Verification items for this drawing (mm, ordinates from the low corner). Round coordinates to 2 decimals unless told otherwise and drop trailing zeros. Loops run counter-clockwise (first coordinate to the right, second up) from the corner with the lowest first, then second, coordinate; pieces in that order, holes last. Notation, with made-up numbers: (72, 8.5) - (122, 8.5) arc R30 cw to (122, 32.5) - close; hole circle Ø5 at (29, -11.75). An arc over 180 degrees is marked (long way). Answer in a Markdown table with one row per item. Add a question column.
(1) Cross-section at A-A on x = 1284.5. Enter the section's corners in (y, z), then the cut area to 3 significant figures.
(2) Cross-section at C-C on y = 37. Enter the section's corners in (x, z).
(3) Thickness scan on line 1 along Z through (x, y) = (1755, 32); line 2 along X through (y, z) = (31, 440). Record the ranges inside material, lowest first.
(4) Cross-section at B-B on z = 305.5. Enter the section's corners in (x, y).
(5) Cross-section at D-D on x = 310. Enter the section's corners in (y, z).
(6) Gauge pin test, flat ends, axial feed: pin 1 (12.5 mm diameter, centred on x = 299.5, y = 18.5, fed in from -Z); pin 2 (7.5 mm diameter, centred on y = 14, z = 964.5, fed in from +X); pin 3 (12.5 mm diameter, centred on y = 8, z = 961, fed in from -X). Record the tip position at first contact, or that the pin passes through.
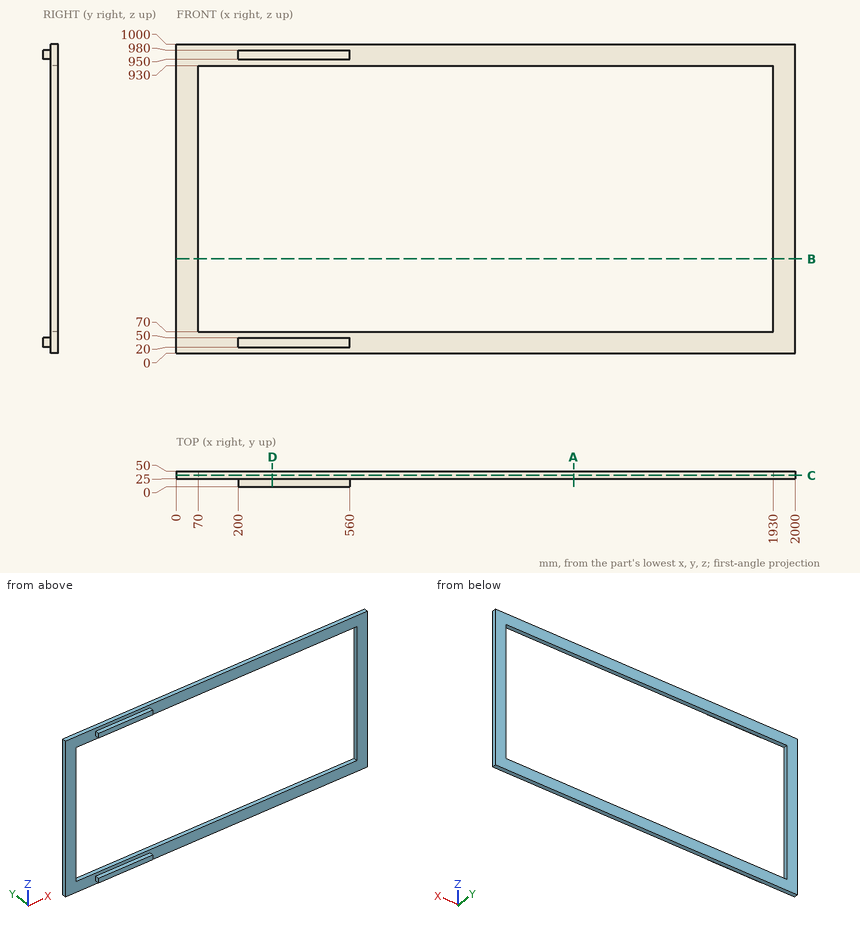
Answers:
| question | item | result |
|---|---|---|
| 1 | outline | (25, 0) - (50, 0) - (50, 70) - (25, 70) - close; (25, 930) - (50, 930) - (50, 1000) - (25, 1000) - close |
| 1 | area | 3,500 mm^2 |
| 2 | outline | (0, 0) - (2000, 0) - (2000, 1000) - (0, 1000) - close; hole (70, 70) - (1930, 70) - (1930, 930) - (70, 930) - close |
| 3 | line 1 | z = 0 to 70, 930 to 1000 |
| 3 | line 2 | x = 0 to 70, 1930 to 2000 |
| 4 | outline | (0, 25) - (70, 25) - (70, 50) - (0, 50) - close; (1930, 25) - (2000, 25) - (2000, 50) - (1930, 50) - close |
| 5 | outline | (0, 20) - (25, 20) - (25, 0) - (50, 0) - (50, 70) - (25, 70) - (25, 50) - (0, 50) - close; (0, 950) - (25, 950) - (25, 930) - (50, 930) - (50, 1000) - (25, 1000) - (25, 980) - (0, 980) - close |
| 6 | pin 1 | stops at z = 20 |
| 6 | pin 2 | stops at x = 560 |
| 6 | pin 3 | stops at x = 200 |
